```python
from build123d import *

# Parameters (mm, degrees)
SKETCH_1_W          = 10
SKETCH_1_H          = 10
EXTRUDE_1_DEPTH     = 1
SKETCH_2_W          = 1.5
SKETCH_2_H          = 0.5
EXTRUDE_2_DEPTH     = 8
CUT_EXTRUDE_2_DEPTH = 2
SKETCH_4_R          = 0.6
CUT_EXTRUDE_3_DEPTH = 2


with BuildPart() as part:
    # 草图1 → 凸台-拉伸1 (new body)
    with BuildSketch(Plane(origin=(0, 0, 0), x_dir=(0, 0, -1), z_dir=(1, 0, 0))):
        with Locations((5, 5)):
            Rectangle(SKETCH_1_W, SKETCH_1_H)
    extrude(amount=EXTRUDE_1_DEPTH)

    # 草图2 → 凸台-拉伸2 (add)
    with BuildSketch(Plane(origin=(1, 0, 0), x_dir=(0, 0, -1), z_dir=(1, 0, 0))):
        with Locations((5, 5)):
            Rectangle(SKETCH_2_W, SKETCH_2_H)
    extrude(amount=EXTRUDE_2_DEPTH)

    # 草图3 → 切除-拉伸2 (cut)
    with BuildSketch(Plane.XZ.offset(-4.75)):
        with BuildLine():
            Line((9, -4.25), (4, -4.25))
            ThreePointArc((4, -4.25), (4.75, -5), (4, -5.75))
            Line((4, -5.75), (9, -5.75))
            Line((9, -5.75), (9, -4.25))
        make_face()
    extrude(amount=-CUT_EXTRUDE_2_DEPTH, mode=Mode.SUBTRACT)

    # 草图4 → 切除-拉伸3 (cut)
    with BuildSketch(Plane.XZ.offset(-4.75)):
        with Locations(Location((4, -5, 0), (0, 0, 270))):
            Circle(SKETCH_4_R)
    extrude(amount=-CUT_EXTRUDE_3_DEPTH, mode=Mode.SUBTRACT)


solid = part.part
```
Here's how the part is built. I have some questions about the finished solid (model axes, mm). A direction names the side the tool comes from. Give positions to 0.01 mm unless a question says otherwise; leave off trailing zeros. Write each loop counter-clockwise with the first axis right and the second up, starting at its lowest first coordinate (ties: lowest second). Pieces come first, ordered by that corner, then holes. Notation, with made-up numbers: (32, -29.5) -> (78, -29.5) arc R4 ccw to (78, -25.5) -> close; hole circle Ø1 at (88.5, -8.5). An arc over 180 degrees is marked (long way). Use one line per item in the form item = value.
1) If I drill on L1, parallel to X at y = 2.25, z = -6.25, over which ranges is the centre line in solid material (lowest first)? Write a range as [from, to].
Verdict:
L1 = [0, 1]
2) On a 3-axis mill with a long thin cutter (end or side, diameter ignored), from which of +Z, -Z, +X, -X, +Y, -Y can I reach the whole of each face in a straight line? I mean faces 1 (the face through (2, 4.75, -5)), 2 (the face through (0.5, 0, -4.9)). Say none if no direction works.
Verdict:
face_1 = +Z, -Z, +X, -Y
face_2 = +Z, -Z, +X, -X, -Y
3) Suppose I cut it at A-A (z = -5). Please give me the cut outline in (x, y).
Verdict:
outline = (0, 0) -> (1, 0) -> (1, 4.75) -> (3.4, 4.75) -> (3.4, 5.25) -> (1, 5.25) -> (1, 10) -> (0, 10) -> close; (4.6, 4.75) -> (4.75, 4.75) -> (4.75, 5.25) -> (4.6, 5.25) -> close
4) Suppose I cut it at B-B (x = 1.8). Please give me the cut outline in (y, z).
Verdict:
outline = (4.75, -5.75) -> (5.25, -5.75) -> (5.25, -4.25) -> (4.75, -4.25) -> close
5) We'd pull the mould along Z, two halves only. Please class faces 3 (the face through (0.5, 4.9, 0)), 4 (the face through (4, 5, -4.4)), 5 (the face through (2, 5.25, -5)): +Z half, -Z half, draft (parallel to the pull), parting line (faces both ways), or undercut.
Verdict:
face_3 = +Z half
face_4 = undercut
face_5 = draft
6) I'm going to push flat-ended pins straight in: pin 1 (1.6 mm diameter, centred on x = 2, z = -5, fed in from -Y); pin 2 (1.6 mm diameter, centred on x = 4, z = -5, fed in from +Y); pin 3 (2 mm diameter, centred on y = 3.5, z = -7.5, fed in from +X). Where does each tip first touch, or does it pass through?
Verdict:
pin_1 = 4.75
pin_2 = 5.25
pin_3 = 1
7) Suppose I cut it at C-C (y = 4.5). Please give me the cut outline in (x, z).
Verdict:
outline = (0, -10) -> (1, -10) -> (1, 0) -> (0, 0) -> close
